Input: part model. Units: mm. Frame: model coordinates. Face numbers are marked on the shaded views. A direction names the side the tool comes from. Round coordinates to 2 decimals unless told otherwise and drop trailing zeros. Loops run counter-clockwise (first coordinate to the right, second up) from the corner with the lowest first, then second, coordinate; pieces in that order, holes last.
(1) Draft query along Z for the marked faces 4, 5, 6 and 7. Return one class per face: released by +Z, released by -Z, zero draft, split by the parting line, or undercut.
(2) Cut plane C-C, the plane z = -16. Output: boundary loops of the cut face in (x, y), and give its area (3 significant figures).
(3) Cut plane B-B, the plane x = 0. Output: boundary loops of the cut face in (y, z), and give its area (3 significant figures).
(4) Access query for the marked faces 1, 2 and 3. Directions: +Z, -Z, +X, -X, +Y, -Y. A direction counts if a zero-diameter tool reaches every point of the face in a straight line with its end or side. Return the directions, or none.
(5) First-contact query: pin 1 Ø1.5 at (x, y) = (6.5, -1) entering from -Z; pin 2 Ø10 at (x, z) = (11, 14.5) entering from -Y; pin 3 Ø3 at (y, z) = (-3, 7.5) entering from +X; pin 4 Ø3 at (x, y) = (-5, -0.5) entering from -Z. Flat tips, straight axial feed; report the tip coordinate or a pass-through.
(6) Cut plane A-A, the plane z = 0. Output: boundary loops of the cut face in (x, y), and give its area (3 significant figures).
(7) Line query: line 1 (X direction, y = 1.5, z = 0); line 2 (Z direction, x = 15.5, y = 2.5). Output: solid intervals per line, ascending.
(8) Cut plane D-D, the plane x = -13. Output: boundary loops of the cut face in (y, z), and give its area (3 significant figures).
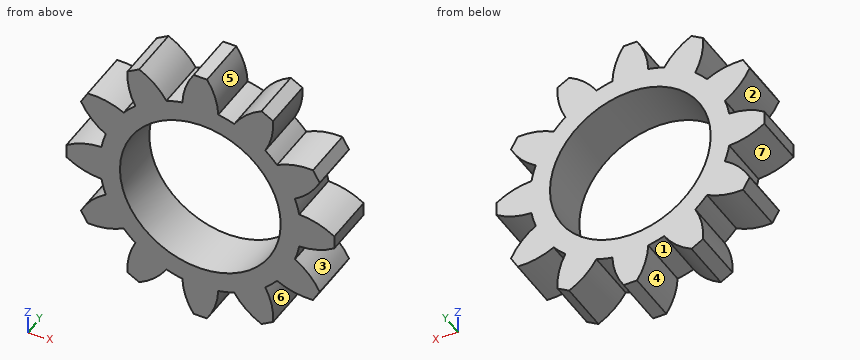
from build123d import *

# Parameters (mm, degrees)
SKETCH1_R           = 12
BOSS_EXTRUDE1_DEPTH = 4


with BuildPart() as part:
    # Sketch1 → Boss-Extrude1 (new body, symmetric)
    with BuildSketch(Plane(origin=(0, 0, 0), x_dir=(1, 0, 0), z_dir=(0, 1, 0))):
        with BuildLine():
            Line((-1, 20), (1, 20))
            ThreePointArc((1, 20), (2.204975942, 17.497232023), (2.675, 14.759551992))
            ThreePointArc((2.675, 14.759551992), (3.882285677, 14.488887394), (5.063158041, 14.119646973))
            ThreePointArc((5.063158041, 14.119646973), (6.839050831, 16.255535399), (9.133974596, 17.820508076))
            Line((9.133974596, 17.820508076), (10.866025404, 16.820508076))
            ThreePointArc((10.866025404, 16.820508076), (10.658181192, 14.050559457), (9.696393951, 11.444646973))
            ThreePointArc((9.696393951, 11.444646973), (10.606601718, 10.606601718), (11.444646973, 9.696393951))
            ThreePointArc((11.444646973, 9.696393951), (14.050559457, 10.658181192), (16.820508076, 10.866025404))
            Line((16.820508076, 10.866025404), (17.820508076, 9.133974596))
            ThreePointArc((17.820508076, 9.133974596), (16.255535399, 6.839050831), (14.119646973, 5.063158041))
            ThreePointArc((14.119646973, 5.063158041), (14.488887394, 3.882285677), (14.759551992, 2.675))
            ThreePointArc((14.759551992, 2.675), (17.497232023, 2.204975942), (20, 1))
            Line((20, 1), (20, -1))
            ThreePointArc((20, -1), (17.497232023, -2.204975942), (14.759551992, -2.675))
            ThreePointArc((14.759551992, -2.675), (14.488887394, -3.882285677), (14.119646973, -5.063158041))
            ThreePointArc((14.119646973, -5.063158041), (16.255535399, -6.839050831), (17.820508076, -9.133974596))
            Line((17.820508076, -9.133974596), (16.820508076, -10.866025404))
            ThreePointArc((16.820508076, -10.866025404), (14.050559457, -10.658181192), (11.444646973, -9.696393951))
            ThreePointArc((11.444646973, -9.696393951), (10.606601718, -10.606601718), (9.696393951, -11.444646973))
            ThreePointArc((9.696393951, -11.444646973), (10.658181192, -14.050559457), (10.866025404, -16.820508076))
            Line((10.866025404, -16.820508076), (9.133974596, -17.820508076))
            ThreePointArc((9.133974596, -17.820508076), (6.839050831, -16.255535399), (5.063158041, -14.119646973))
            ThreePointArc((5.063158041, -14.119646973), (3.882285677, -14.488887394), (2.675, -14.759551992))
            ThreePointArc((2.675, -14.759551992), (2.204975942, -17.497232023), (1, -20))
            Line((1, -20), (-1, -20))
            ThreePointArc((-1, -20), (-2.204975942, -17.497232023), (-2.675, -14.759551992))
            ThreePointArc((-2.675, -14.759551992), (-3.882285677, -14.488887394), (-5.063158041, -14.119646973))
            ThreePointArc((-5.063158041, -14.119646973), (-6.839050831, -16.255535399), (-9.133974596, -17.820508076))
            Line((-9.133974596, -17.820508076), (-10.866025404, -16.820508076))
            ThreePointArc((-10.866025404, -16.820508076), (-10.658181192, -14.050559457), (-9.696393951, -11.444646973))
            ThreePointArc((-9.696393951, -11.444646973), (-10.606601718, -10.606601718), (-11.444646973, -9.696393951))
            ThreePointArc((-11.444646973, -9.696393951), (-14.050559457, -10.658181192), (-16.820508076, -10.866025404))
            Line((-16.820508076, -10.866025404), (-17.820508076, -9.133974596))
            ThreePointArc((-17.820508076, -9.133974596), (-16.255535399, -6.839050831), (-14.119646973, -5.063158041))
            ThreePointArc((-14.119646973, -5.063158041), (-14.488887394, -3.882285677), (-14.759551992, -2.675))
            ThreePointArc((-14.759551992, -2.675), (-17.497232023, -2.204975942), (-20, -1))
            Line((-20, -1), (-20, 1))
            ThreePointArc((-20, 1), (-17.497232023, 2.204975942), (-14.759551992, 2.675))
            ThreePointArc((-14.759551992, 2.675), (-14.488887394, 3.882285677), (-14.119646973, 5.063158041))
            ThreePointArc((-14.119646973, 5.063158041), (-16.255535399, 6.839050831), (-17.820508076, 9.133974596))
            Line((-17.820508076, 9.133974596), (-16.820508076, 10.866025404))
            ThreePointArc((-16.820508076, 10.866025404), (-14.050559457, 10.658181192), (-11.444646973, 9.696393951))
            ThreePointArc((-11.444646973, 9.696393951), (-10.606601718, 10.606601718), (-9.696393951, 11.444646973))
            ThreePointArc((-9.696393951, 11.444646973), (-10.658181192, 14.050559457), (-10.866025404, 16.820508076))
            Line((-10.866025404, 16.820508076), (-9.133974596, 17.820508076))
            ThreePointArc((-9.133974596, 17.820508076), (-6.839050831, 16.255535399), (-5.063158041, 14.119646973))
            ThreePointArc((-5.063158041, 14.119646973), (-3.882285677, 14.488887394), (-2.675, 14.759551992))
            ThreePointArc((-2.675, 14.759551992), (-2.204975942, 17.497232023), (-1, 20))
        make_face()
        Circle(SKETCH1_R, mode=Mode.SUBTRACT)
    extrude(amount=BOSS_EXTRUDE1_DEPTH, both=True)


solid = part.part
Reported:
1. face 4: released by -Z
1. face 5: released by +Z
1. face 6: undercut
1. face 7: undercut
2. outline: (-10.89, -4) - (-6.57, -4) - (-6.57, 4) - (-10.89, 4) - close; (-2.56, -4) - (2.56, -4) - (2.56, 4) - (-2.56, 4) - close; (6.57, -4) - (10.89, -4) - (10.89, 4) - (6.57, 4) - close
2. area: 110 mm2
3. outline: (-4, -20) - (4, -20) - (4, -12) - (-4, -12) - close; (-4, 12) - (4, 12) - (4, 20) - (-4, 20) - close
3. area: 128 mm2
4. face 1: -Z, +Y, -Y
4. face 2: -X, +Y, -Y
4. face 3: +X, +Y, -Y
5. pin 1: stops at z = -16.61
5. pin 2: stops at y = -4
5. pin 3: stops at x = 17.75
5. pin 4: stops at z = -15.93
6. outline: (-20, -4) - (-12, -4) - (-12, 4) - (-20, 4) - close; (12, -4) - (20, -4) - (20, 4) - (12, 4) - close
6. area: 128 mm2
7. line 1: x = -20 to -12, 12 to 20
7. line 2: z = -10.86 to -6.09, -2.62 to 2.62, 6.09 to 10.86
8. outline: (-4, -10.37) - (4, -10.37) - (4, 10.37) - (-4, 10.37) - close
8. area: 166 mm2
